Work out the finished part from the listing and answer in its coordinate system (mm). Face numbers are marked on the shaded views. A direction names the side the tool comes from. Round coordinates to 2 decimals unless told otherwise and drop trailing zeros. Loops run counter-clockwise (first coordinate to the right, second up) from the corner with the lowest first, then second, coordinate; pieces in that order, holes last. Notation, with made-up numbers: M 49.5,74.5 L 93.5,74.5 A10 ccw 93.5,80.5 Z; hole C -27,56 d11. An arc over 180 degrees is marked long. One line per item, written item: value.
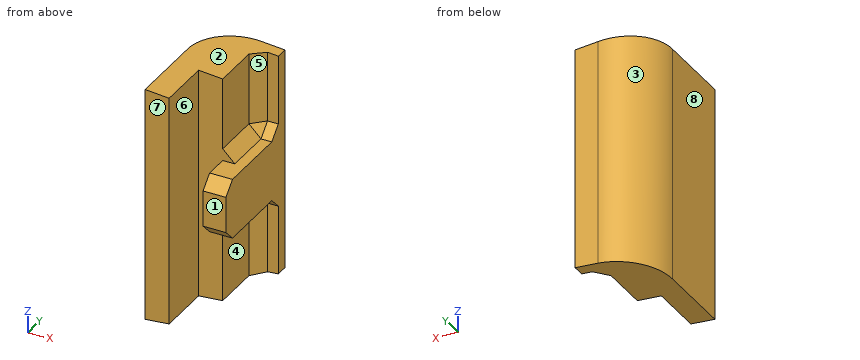
```python
from build123d import *

# Parameters (mm, degrees)
BOSS_EXTRUDE1_START       = -62.152648455
BOSS_EXTRUDE1_DEPTH       = 62.152648455
BOSS_EXTRUDE1_START_2     = 33.419354119
BOSS_EXTRUDE1_2_OUTLINE_W = 41
BOSS_EXTRUDE1_2_OUTLINE_H = 70
BOSS_EXTRUDE1_2_DEPTH     = 4.580645881
SKETCH2_W                 = 31.75
SKETCH2_H                 = 50.8
BOSS_EXTRUDE2_DEPTH       = 12.035499154
CHAMFER1_SIZE             = 6.35


with BuildPart() as part:
    # Boss-Extrude1: read off the stored shape, not the designer's step
    # Boss-Extrude1 outline → Boss-Extrude1 (new body)
    with BuildSketch(Plane.XY.offset(BOSS_EXTRUDE1_START)):
        with BuildLine():
            Line((-301.612263914, 87.858595148), (-289.57676476, 87.858595148))
            Line((-289.57676476, 87.858595148), (-289.57676476, 94.208595148))
            Line((-289.57676476, 94.208595148), (-301.56393658, 94.208595148))
            ThreePointArc((-301.56393658, 94.208595148), (-319.524448822, 86.76910739), (-326.96393658, 68.808595148))
            Line((-326.96393658, 68.808595148), (-326.96393658, 27.533595148))
            Line((-326.96393658, 27.533595148), (-314.312263914, 27.533595148))
            Line((-314.312263914, 27.533595148), (-314.312263914, 56.108595148))
            Line((-314.312263914, 56.108595148), (-301.612263914, 56.108595148))
            Line((-301.612263914, 56.108595148), (-301.612263914, 87.858595148))
        make_face()
    boss_extrude1 = extrude(amount=BOSS_EXTRUDE1_DEPTH)

    # Boss-Extrude1 2 outline → Boss-Extrude1 2 (cut)
    with BuildSketch(Plane(origin=(0, 0, 0), x_dir=(0.9961946980917454, 0, 0.08715574274765814), z_dir=(0.08715574274765815, 0, -0.9961946980917455)).offset(BOSS_EXTRUDE1_START_2)):
        with Locations((-312.5, -61)):
            Rectangle(BOSS_EXTRUDE1_2_OUTLINE_W, BOSS_EXTRUDE1_2_OUTLINE_H)
    boss_extrude1_2 = extrude(amount=BOSS_EXTRUDE1_2_DEPTH, mode=Mode.SUBTRACT)

    # Mirror1: Boss-Extrude1, Boss-Extrude1 2 across plane
    add(boss_extrude1.mirror(Plane.XY))
    add(boss_extrude1_2.mirror(Plane.XY), mode=Mode.SUBTRACT)

    # Sketch2 → Boss-Extrude2 (add)
    with BuildSketch(Plane(origin=(-301.612263914, 0, 0), x_dir=(0, 0, -1), z_dir=(1, 0, 0))):
        with Locations((0, 62.458595148)):
            Rectangle(SKETCH2_W, SKETCH2_H)
    extrude(amount=BOSS_EXTRUDE2_DEPTH)

    # Chamfer1
    chamfer1_edges = [part.edges().sort_by_distance(p)[0] for p in [
        (-295.594514337, 37.058595148, -15.875),
        (-295.594514337, 37.058595148, 15.875),
        (-295.594514337, 87.858595148, 15.875),
        (-301.612263914, 87.858595148, 37.904832248),
        (-301.612263914, 71.983595148, 15.875),
        (-295.594514337, 87.858595148, -15.875),
        (-301.612263914, 71.983595148, -15.875),
        (-301.612263914, 87.858595148, -37.904832248),
    ]]
    chamfer(chamfer1_edges, length=CHAMFER1_SIZE)


solid = part.part
```
1) Find section D-D (x = -293). Give the vertices of the cut face in (y, z) (3 decimals).
Check values:
outline: M 37.059,-9.525 L 43.409,-15.875 L 81.509,-15.875 L 87.859,-22.225 L 87.859,-59.181 L 94.209,-59.181 L 94.209,59.181 L 87.859,59.181 L 87.859,22.225 L 81.509,15.875 L 43.409,15.875 L 37.059,9.525 Z
2) Find section A-A (y = 51). Give the vertices of the cut face in (x, z) (3 decimals), then the cut area to 3 significant figures.
Check values:
outline: M -326.964,-62.153 L -314.312,-61.046 L -314.312,61.046 L -326.964,62.153 Z; M -301.612,-15.875 L -289.577,-15.875 L -289.577,15.875 L -301.612,15.875 Z
area: 1,940 mm2
3) For the marked faces 1, 2, 3, 4 and 5, determine the directions among +Z, -Z, +X, -X, +Y, -Y from which every point of the face is accessible in a straight line to the end or side of a thin tool.
Check values:
face 1: +Z, -Z, +X, -Y
face 2: +Z, +X, +Y, -Y
face 3: +Z, -Z, -X, +Y
face 4: -Z, +X, -Y
face 5: +Z, +X, -Y
4) Each of these flat-tipped pins is pushed along its axis until it touches: pin 1 (4 mm diameter, centred on x = -320, z = -38.5, fed in from +Y); pin 2 (9.5 mm diameter, centred on x = -304.5, z = -10, fed in from -Y); pin 3 (2 mm diameter, centred on y = 78, z = 47, fed in from +X). Where does it stop, or does it pass through?
Check values:
pin 1: y = 88.17
pin 2: y = 37.06
pin 3: x = -301.61
5) Find section C-C (y = 66). Give the vertices of the cut face in (x, z) (3 decimals), then the cut area to 3 significant figures.
Check values:
outline: M -326.964,-62.153 L -301.612,-59.935 L -301.612,-22.225 L -295.262,-15.875 L -289.577,-15.875 L -289.577,15.875 L -295.262,15.875 L -301.612,22.225 L -301.612,59.935 L -326.964,62.153 Z
area: 3,520 mm2
6) Find the intervals of material crossed by probe 1 along Y at (x, z) = (-295, -36); probe 2 along X at (y, z) = (36, -30.5); probe 3 along Z at (x, y) = (-292, 63) (3 decimals), in increasing order. Write a range as from..to.
Check values:
probe 1: 87.86..94.21
probe 2: -326.96..-314.31
probe 3: -15.875..15.875
7) The mould has two halves that part along X. Classify the marked faces 6, 7 and 8: +X half, -X half, draft (parallel to the pull), parting line (faces both ways), or undercut.
Check values:
face 6: undercut
face 7: draft
face 8: -X half
8) Find section B-B (z = -38). Give the vertices of the cut face in (x, y), then the cut area to 3 significant figures.
Check values:
outline: M -326.96,27.53 L -314.31,27.53 L -314.31,56.11 L -301.61,56.11 L -301.61,81.51 L -295.26,87.86 L -289.58,87.86 L -289.58,94.21 L -301.56,94.21 A25.4 ccw -326.96,68.81 Z
area: 1,290 mm2
